Build history of the part. All positions in model axes, mm. A direction names the side the tool comes from. Round coordinates to 2 decimals unless told otherwise and drop trailing zeros. One line per item, written item: value.
```python
from build123d import *

# Parameters (mm, degrees)
SKETCH1_R           = 6
SKETCH1_R_2         = 3
BOSS_EXTRUDE1_DEPTH = 560


with BuildPart() as part:
    # Sketch1 → Boss-Extrude1 (new body)
    with BuildSketch(Plane(origin=(0, 0, 0), x_dir=(0, 0, -1), z_dir=(1, 0, 0))):
        with BuildLine():
            Line((-20, -4), (-17, -4))
            Line((-17, -4), (-17, -10))
            Line((-17, -10), (-13, -10))
            Line((-13, -10), (-8.5, -5.5))
            Line((-8.5, -5.5), (-8.5, 5.5))
            Line((-8.5, 5.5), (-13, 10))
            Line((-13, 10), (-17, 10))
            Line((-17, 10), (-17, 4))
            Line((-17, 4), (-20, 4))
            Line((-20, 4), (-20, 36))
            Line((-20, 36), (-17, 36))
            Line((-17, 36), (-17, 30))
            Line((-17, 30), (-13, 30))
            Line((-13, 30), (-8.5, 34.5))
            Line((-8.5, 34.5), (-8.5, 45.5))
            Line((-8.5, 45.5), (-13, 50))
            Line((-13, 50), (-17, 50))
            Line((-17, 50), (-17, 44))
            Line((-17, 44), (-20, 44))
            Line((-20, 44), (-20, 57))
            ThreePointArc((-20, 57), (-19.121320344, 59.121320344), (-17, 60))
            Line((-17, 60), (-4, 60))
            Line((-4, 60), (-4, 57))
            Line((-4, 57), (-10, 57))
            Line((-10, 57), (-10, 53))
            Line((-10, 53), (-5.5, 48.5))
            Line((-5.5, 48.5), (5.5, 48.5))
            Line((5.5, 48.5), (10, 53))
            Line((10, 53), (10, 57))
            Line((10, 57), (4, 57))
            Line((4, 57), (4, 60))
            Line((4, 60), (17, 60))
            ThreePointArc((17, 60), (19.121320344, 59.121320344), (20, 57))
            Line((20, 57), (20, 44))
            Line((20, 44), (17, 44))
            Line((17, 44), (17, 50))
            Line((17, 50), (13, 50))
            Line((13, 50), (8.5, 45.5))
            Line((8.5, 45.5), (8.5, 34.5))
            Line((8.5, 34.5), (13, 30))
            Line((13, 30), (17, 30))
            Line((17, 30), (17, 36))
            Line((17, 36), (20, 36))
            Line((20, 36), (20, 20))
            Line((20, 20), (20, 4))
            Line((20, 4), (17, 4))
            Line((17, 4), (17, 10))
            Line((17, 10), (13, 10))
            Line((13, 10), (8.5, 5.5))
            Line((8.5, 5.5), (8.5, -5.5))
            Line((8.5, -5.5), (13, -10))
            Line((13, -10), (17, -10))
            Line((17, -10), (17, -4))
            Line((17, -4), (20, -4))
            Line((20, -4), (20, -17))
            ThreePointArc((20, -17), (19.121320344, -19.121320344), (17, -20))
            Line((17, -20), (4, -20))
            Line((4, -20), (4, -17))
            Line((4, -17), (10, -17))
            Line((10, -17), (10, -13))
            Line((10, -13), (5.5, -8.5))
            Line((5.5, -8.5), (-5.5, -8.5))
            Line((-5.5, -8.5), (-10, -13))
            Line((-10, -13), (-10, -17))
            Line((-10, -17), (-4, -17))
            Line((-4, -17), (-4, -20))
            Line((-4, -20), (-17, -20))
            ThreePointArc((-17, -20), (-19.121320344, -19.121320344), (-20, -17))
            Line((-20, -17), (-20, -4))
        make_face()
        Circle(SKETCH1_R, mode=Mode.SUBTRACT)
        with Locations((-15, -15)):
            Circle(SKETCH1_R_2, mode=Mode.SUBTRACT)
        with Locations((15, 55)):
            Circle(SKETCH1_R_2, mode=Mode.SUBTRACT)
        with Locations((-15, 55)):
            Circle(SKETCH1_R_2, mode=Mode.SUBTRACT)
        with Locations((15, -15)):
            Circle(SKETCH1_R_2, mode=Mode.SUBTRACT)
        with Locations((0, 40)):
            Circle(SKETCH1_R, mode=Mode.SUBTRACT)
        Polygon((-5.5, 8.5), (-17, 20), (-5.5, 31.5), (5.5, 31.5), (17, 20), (5.5, 8.5), align=None, mode=Mode.SUBTRACT)
    extrude(amount=BOSS_EXTRUDE1_DEPTH)


solid = part.part
```
Item 1: Which spindle directions (+Z, -Z, +X, -X, +Y, -Y) get a long thin tool onto all of the face, cutting with end or side? Do faces 1 (the face through (276, 48.5, 0)), 2 (the face through (276, 20, -20)). Say none if no direction does.
Check values:
face 1: +X, -X
face 2: -Z, +X, -X, +Y, -Y
Item 2: Slice it at A-A, the plane x = 469.5. Give the number of separate pieces and of enclosed holes in the cut face, and give its area (3 significant figures).
Check values:
separate pieces: 1
enclosed holes: 7
area: 1,290 mm2
Item 3: Wall check: line 1 along Y through (x, z) = (143, 0); line 2 along Z through (x, y) = (98, 37.5); line 3 along Z through (x, y) = (202, 28.5). Give the ranges that are in metal, low to high.
Check values:
line 1: y = -8.5 to -6, 6 to 8.5, 31.5 to 34, 46 to 48.5
line 2: z = -8.5 to -5.45, 5.45 to 8.5
line 3: z = -20 to -8.5, 8.5 to 20
Item 4: Pull direction Z, two halves, no side cores. Call faces 3 (the face through (276, -11, 20)), 4 (the face through (276, 14, -11)), 5 (the face through (276, 51, -20)), 6 (the face through (276, 8.5, 0)): pulls with the +Z half, pulls with the -Z half, needs draft (parallel to the pull), parting line crosses it, or undercut.
Check values:
face 3: pulls with the +Z half
face 4: undercut
face 5: pulls with the -Z half
face 6: undercut
Item 5: Drop a flat-ended pin along its axis: P1, Ø3.5, axis at x = 293, z = 0.5, coming from the +Y side. Give the stop position or say it passes through.
Check values:
P1: stops at y = 48.5
